from build123d import *

# Parameters (mm, degrees)
BOSS_EXTRUDE1_DEPTH = 12


with BuildPart() as part:
    # Sketch1 → Boss-Extrude1 (new body)
    with BuildSketch(Plane.XY):
        with BuildLine():
            Line((-398.481522137, 104.896883683), (-351.779111417, 104.896883683))
            ThreePointArc((-351.779111417, 104.896883683), (-348.011442278, 104.39201543), (-348.481522137, 108.164182926))
            Line((-348.481522137, 108.164182926), (-348.481522137, 116.896883683))
            Line((-348.481522137, 116.896883683), (-298.481522137, 116.896883683))
            Line((-298.481522137, 116.896883683), (-298.481522137, 108.164182926))
            ThreePointArc((-298.481522137, 108.164182926), (-298.951601996, 104.39201543), (-295.183932857, 104.896883683))
            Line((-295.183932857, 104.896883683), (-251.779111417, 104.896883683))
            ThreePointArc((-251.779111417, 104.896883683), (-248.011442278, 104.39201543), (-248.481522137, 108.164182926))
            Line((-248.481522137, 108.164182926), (-248.481522137, 116.896883683))
            Line((-248.481522137, 116.896883683), (-198.481522137, 116.896883683))
            Line((-198.481522137, 116.896883683), (-198.481522137, 108.164182926))
            ThreePointArc((-198.481522137, 108.164182926), (-198.951601996, 104.39201543), (-195.183932857, 104.896883683))
            Line((-195.183932857, 104.896883683), (-151.779111417, 104.896883683))
            ThreePointArc((-151.779111417, 104.896883683), (-148.011442278, 104.39201543), (-148.481522137, 108.164182926))
            Line((-148.481522137, 108.164182926), (-148.481522137, 116.896883683))
            Line((-148.481522137, 116.896883683), (-98.481522137, 116.896883683))
            Line((-98.481522137, 116.896883683), (-98.481522137, 108.164182926))
            ThreePointArc((-98.481522137, 108.164182926), (-98.951601996, 104.39201543), (-95.183932857, 104.896883683))
            Line((-95.183932857, 104.896883683), (-51.779111417, 104.896883683))
            ThreePointArc((-51.779111417, 104.896883683), (-48.011442278, 104.39201543), (-48.481522137, 108.164182926))
            Line((-48.481522137, 108.164182926), (-48.481522137, 116.896883683))
            Line((-48.481522137, 116.896883683), (1.518477863, 116.896883683))
            Line((1.518477863, 116.896883683), (1.518477863, 108.164182926))
            ThreePointArc((1.518477863, 108.164182926), (1.048398004, 104.39201543), (4.816067143, 104.896883683))
            Line((4.816067143, 104.896883683), (48.220888583, 104.896883683))
            ThreePointArc((48.220888583, 104.896883683), (51.988557722, 104.39201543), (51.518477863, 108.164182926))
            Line((51.518477863, 108.164182926), (51.518477863, 116.896883683))
            Line((51.518477863, 116.896883683), (101.518477863, 116.896883683))
            Line((101.518477863, 116.896883683), (101.518477863, 108.164182926))
            ThreePointArc((101.518477863, 108.164182926), (101.048398004, 104.39201543), (104.816067143, 104.896883683))
            Line((104.816067143, 104.896883683), (148.220888583, 104.896883683))
            ThreePointArc((148.220888583, 104.896883683), (151.988557722, 104.39201543), (151.518477863, 108.164182926))
            Line((151.518477863, 108.164182926), (151.518477863, 116.896883683))
            Line((151.518477863, 116.896883683), (176.518477863, 116.896883683))
            Line((176.518477863, 116.896883683), (176.518477863, 108.164182926))
            ThreePointArc((176.518477863, 108.164182926), (176.048398004, 104.39201543), (179.816067143, 104.896883683))
            Line((179.816067143, 104.896883683), (223.220888583, 104.896883683))
            ThreePointArc((223.220888583, 104.896883683), (226.988557722, 104.39201543), (226.518477863, 108.164182926))
            Line((226.518477863, 108.164182926), (226.518477863, 116.896883683))
            Line((226.518477863, 116.896883683), (276.518477863, 116.896883683))
            Line((276.518477863, 116.896883683), (276.518477863, 108.164182926))
            ThreePointArc((276.518477863, 108.164182926), (276.048398004, 104.39201543), (279.816067143, 104.896883683))
            Line((279.816067143, 104.896883683), (323.220888583, 104.896883683))
            ThreePointArc((323.220888583, 104.896883683), (326.988557722, 104.39201543), (326.518477863, 108.164182926))
            Line((326.518477863, 108.164182926), (326.518477863, 116.896883683))
            Line((326.518477863, 116.896883683), (376.518477863, 116.896883683))
            Line((376.518477863, 116.896883683), (376.518477863, 108.164182926))
            ThreePointArc((376.518477863, 108.164182926), (376.048398004, 104.39201543), (379.816067143, 104.896883683))
            Line((379.816067143, 104.896883683), (423.220888583, 104.896883683))
            ThreePointArc((423.220888583, 104.896883683), (426.988557722, 104.39201543), (426.518477863, 108.164182926))
            Line((426.518477863, 108.164182926), (426.518477863, 116.896883683))
            Line((426.518477863, 116.896883683), (476.518477863, 116.896883683))
            Line((476.518477863, 116.896883683), (476.518477863, 108.164182926))
            ThreePointArc((476.518477863, 108.164182926), (476.048398004, 104.39201543), (479.816067143, 104.896883683))
            Line((479.816067143, 104.896883683), (523.220888583, 104.896883683))
            ThreePointArc((523.220888583, 104.896883683), (526.988557722, 104.39201543), (526.518477863, 108.164182926))
            Line((526.518477863, 108.164182926), (526.518477863, 116.896883683))
            Line((526.518477863, 116.896883683), (576.518477863, 116.896883683))
            Line((576.518477863, 116.896883683), (576.518477863, 108.164182926))
            ThreePointArc((576.518477863, 108.164182926), (576.048398004, 104.39201543), (579.816067143, 104.896883683))
            Line((579.816067143, 104.896883683), (623.220888583, 104.896883683))
            ThreePointArc((623.220888583, 104.896883683), (626.988557722, 104.39201543), (626.518477863, 108.164182926))
            Line((626.518477863, 108.164182926), (626.518477863, 116.896883683))
            Line((626.518477863, 116.896883683), (676.518477863, 116.896883683))
            Line((676.518477863, 116.896883683), (676.518477863, 108.164182926))
            ThreePointArc((676.518477863, 108.164182926), (676.048398004, 104.39201543), (679.816067143, 104.896883683))
            Line((679.816067143, 104.896883683), (726.518477863, 104.896883683))
            Line((726.518477863, 104.896883683), (726.518477863, 57.896883683))
            Line((726.518477863, 57.896883683), (717.793597981, 57.896883683))
            ThreePointArc((717.793597981, 57.896883683), (714.01671802, 58.392576145), (714.518477863, 54.616497449))
            Line((714.518477863, 54.616497449), (714.518477863, 14.177269917))
            ThreePointArc((714.518477863, 14.177269917), (714.01671802, 10.401191221), (717.793597981, 10.896883683))
            Line((717.793597981, 10.896883683), (726.518477863, 10.896883683))
            Line((726.518477863, 10.896883683), (726.518477863, -36.103116317))
            Line((726.518477863, -36.103116317), (717.793597981, -36.103116317))
            ThreePointArc((717.793597981, -36.103116317), (714.01671802, -35.607423855), (714.518477863, -39.383502551))
            Line((714.518477863, -39.383502551), (714.518477863, -71.103116317))
            Line((714.518477863, -71.103116317), (714.518477863, -83.103116317))
            Line((714.518477863, -83.103116317), (-386.481522137, -83.103116317))
            Line((-386.481522137, -83.103116317), (-386.481522137, -39.383502551))
            ThreePointArc((-386.481522137, -39.383502551), (-385.979762293, -35.607423855), (-389.756642255, -36.103116317))
            Line((-389.756642255, -36.103116317), (-398.481522137, -36.103116317))
            Line((-398.481522137, -36.103116317), (-398.481522137, 10.896883683))
            Line((-398.481522137, 10.896883683), (-389.756642255, 10.896883683))
            ThreePointArc((-389.756642255, 10.896883683), (-385.979762293, 10.401191221), (-386.481522137, 14.177269917))
            Line((-386.481522137, 14.177269917), (-386.481522137, 54.616497449))
            ThreePointArc((-386.481522137, 54.616497449), (-385.979762293, 58.392576145), (-389.756642255, 57.896883683))
            Line((-389.756642255, 57.896883683), (-398.481522137, 57.896883683))
            Line((-398.481522137, 57.896883683), (-398.481522137, 104.896883683))
        make_face()
    extrude(amount=BOSS_EXTRUDE1_DEPTH)


solid = part.part
Part model, mm, in its own coordinate system. Round coordinates to 2 decimals unless told otherwise and drop trailing zeros. Order: outer loops, then holes, each group sorted by start corner. A loop starts at its lowest first (then second) coordinate and runs counter-clockwise, first axis right, second up. Notation, with made-up numbers: (-3.75, 46.25) -> (19.25, 46.25) arc R25 cw to (19.25, 72.25) -> close; hole circle Ø7 at (82.5, 26). An arc over 180 degrees is marked (long way). Put each result on its own line as item: value.
Q1. Pin check, flat tips, straight feed: pin 1 Ø4.5 at (x, z) = (721, 8) entering from +Y; pin 2 Ø2.5 at (y, z) = (110.5, 4.5) entering from +X; pin 3 Ø2.5 at (y, z) = (111.5, 3.5) entering from -X. Stop position of each tip, or through.
From the geometry:
pin 1: stops at y = 104.9
pin 2: stops at x = 676.52
pin 3: stops at x = -348.48
Q2. Wall check: line 1 (X direction, y = 34, z = 7.5); line 2 (Y direction, x = -98, z = 5); line 3 (Y direction, x = 148, z = 6.5). Give the ranges that are in metal, low to high. Write a range as [from, to].
From the geometry:
line 1: x = [-386.48, 714.52]
line 2: y = [-83.1, 103.81]
line 3: y = [-83.1, 104.9]
Q3. Band-saw the part on B-B (x = 203). Give the cut face in (y, z).
From the geometry:
outline: (-83.1, 0) -> (104.9, 0) -> (104.9, 12) -> (-83.1, 12) -> close
Q4. Band-saw the part on A-A (y = 40). Give the cut face in (x, z).
From the geometry:
outline: (-386.48, 0) -> (714.52, 0) -> (714.52, 12) -> (-386.48, 12) -> close
